The listing builds one solid part. Answer for the finished solid, in the listing's coordinates (mm). A direction names the side the tool comes from. Round coordinates to 2 decimals unless told otherwise and drop trailing zeros. Write each loop counter-clockwise with the first axis right and the second up, starting at its lowest first coordinate (ties: lowest second). Pieces come first, ordered by that corner, then holes.
Item 1: Find the intervals of material crossed by probe 1 along Y at (x, z) = (1, 100); probe 2 along Z at (x, y) = (9.5, 0); probe 3 along Z at (x, y) = (-14.5, 26.5), in increasing order.
Item 2: Find section C-C on y = -74. Give the vertices of the cut face in (x, z), then the cut area to 3 significant figures.
Item 3: Each of these flat-tipped pins is pushed along its axis until it touches: pin 1 (10 mm diameter, centred on x = -3.5, z = 108, fed in from +Y); pin 2 (12 mm diameter, centred on x = -8, y = -30.5, fed in from +Z); pin 3 (3 mm diameter, centred on x = -4, z = 196, fed in from -Y). Where does it stop, or does it pass through?
Item 4: A tool of negligible diameter and unlimited length cuts with its end or side. For faces 4 (the face through (0, -9, 204.67)), 5 (the face through (12.492, -188.764, 169.536)), 6 (the face through (16.239, -190.054, 170.824)), 7 (the face through (0, -10, 205.87)), 8 (the face through (-11.95, -186.23, 167.04)), from which of +Z, -Z, +X, -X, +Y, -Y can it reach the whole face along a straight path? Write none if from no direction.
Item 5: For a pull along X with two mould halves and no side action, classify faces 1 (the face through (14.48, -189.95, 170.72)), 2 (the face through (-16.239, -190.908, 171.667)), 3 (the face through (-13.758, -190.633, 171.393)) as +X half, -X half, draft (parallel to the pull), parting line (faces both ways), or undercut.
Item 6: Find section A-A on z = 118. Give the vertices of the cut face in (x, y), then the cut area to 3 significant figures.
Item 7: Find section B-B on x = -5.5. Give the vertices of the cut face in (y, z) (3 decimals), then the cut area to 3 significant figures.
```python
from build123d import *


with BuildPart() as part:
    # 扫描1: sweep along a path in 草图1
    with BuildLine(Plane(origin=(0, 0, 0), x_dir=(0, 0, -1), z_dir=(1, 0, 0))) as sweep_1_path:
        Line((-211.869954442, 132.702101833), (-211.869954442, -150.705045558))
        Line((-211.869954442, -150.705045558), (-132.575, -230))
        Line((-132.575, -230), (-84.915, -230))
    # 草图2 → 扫描1 (sweep)
    with BuildSketch(Plane(origin=(0, 132.702101833, 211.869954442), x_dir=(1, 0, 0), z_dir=(0, 1, 0))):
        with BuildLine():
            Line((17.5, 0), (14.94151844, 0))
            ThreePointArc((14.94151844, 0), (13.772097871, 0.37751563), (13.044151844, 1.367544468))
            Line((13.044151844, 1.367544468), (11.955848156, 4.632455532))
            ThreePointArc((11.955848156, 4.632455532), (11.227902129, 5.62248437), (10.05848156, 6))
            Line((10.05848156, 6), (-10.05848156, 6))
            ThreePointArc((-10.05848156, 6), (-11.227902129, 5.62248437), (-11.955848156, 4.632455532))
            Line((-11.955848156, 4.632455532), (-13.044151844, 1.367544468))
            ThreePointArc((-13.044151844, 1.367544468), (-13.772097871, 0.37751563), (-14.94151844, 0))
            Line((-14.94151844, 0), (-17.5, 0))
            Line((-17.5, 0), (-17.5, 1.2))
            Line((-17.5, 1.2), (-14.94151844, 1.2))
            ThreePointArc((-14.94151844, 1.2), (-14.473750212, 1.351006252), (-14.182571802, 1.747017787))
            Line((-14.182571802, 1.747017787), (-13.094268114, 5.011928851))
            ThreePointArc((-13.094268114, 5.011928851), (-11.929554471, 6.595974993), (-10.05848156, 7.2))
            Line((-10.05848156, 7.2), (10.05848156, 7.2))
            ThreePointArc((10.05848156, 7.2), (11.929554471, 6.595974993), (13.094268114, 5.011928851))
            Line((13.094268114, 5.011928851), (14.182571802, 1.747017787))
            ThreePointArc((14.182571802, 1.747017787), (14.473750212, 1.351006252), (14.94151844, 1.2))
            Line((14.94151844, 1.2), (17.5, 1.2))
            Line((17.5, 1.2), (17.5, 0))
        make_face()
    sweep(path=sweep_1_path.line, transition=Transition.RIGHT)


solid = part.part
```
Check values:
1. probe 1: y = -224 to -222.8
1. probe 2: z = 204.67 to 205.87
1. probe 3: z = 210.54 to 211.82
2. outline: (-17.5, 210.67) - (-14.94, 210.67) arc R0.8 cw to (-14.18, 210.12) - (-13.09, 206.86) arc R3.2 ccw to (-10.06, 204.67) - (10.06, 204.67) arc R3.2 ccw to (13.09, 206.86) - (14.18, 210.12) arc R0.8 cw to (14.94, 210.67) - (17.5, 210.67) - (17.5, 211.87) - (14.94, 211.87) arc R2 ccw to (13.04, 210.5) - (11.96, 207.24) arc R2 cw to (10.06, 205.87) - (-10.06, 205.87) arc R2 cw to (-11.96, 207.24) - (-13.04, 210.5) arc R2 ccw to (-14.94, 211.87) - (-17.5, 211.87) - close
2. area: 50.5 mm2
3. pin 1: stops at y = -222.8
3. pin 2: stops at z = 211.63
3. pin 3: stops at y = -159.59
4. face 4: -Z, +X, -X, +Y
4. face 5: +Z, -Y
4. face 6: -Z, +X, +Y
4. face 7: +Z, +Y, -Y
4. face 8: -Z, -X, +Y
5. face 1: +X half
5. face 2: draft
5. face 3: undercut
6. outline: (-17.5, -230) - (-14.94, -230) arc R2 ccw to (-13.04, -228.63) - (-11.96, -225.37) arc R2 cw to (-10.06, -224) - (10.06, -224) arc R2 cw to (11.96, -225.37) - (13.04, -228.63) arc R2 ccw to (14.94, -230) - (17.5, -230) - (17.5, -228.8) - (14.94, -228.8) arc R0.8 cw to (14.18, -228.25) - (13.09, -224.99) arc R3.2 ccw to (10.06, -222.8) - (-10.06, -222.8) arc R3.2 ccw to (-13.09, -224.99) - (-14.18, -228.25) arc R0.8 cw to (-14.94, -228.8) - (-17.5, -228.8) - close
6. area: 50.5 mm2
7. outline: (-224, 84.915) - (-222.8, 84.915) - (-222.8, 129.593) - (-147.723, 204.67) - (132.702, 204.67) - (132.702, 205.87) - (-148.22, 205.87) - (-224, 130.09) - close
7. area: 519 mm2
